```python
from build123d import *

# Parameters (mm, degrees)
SKETCH_1_W          = 100
SKETCH_1_H          = 5
EXTRUDE_1_DEPTH     = 8.8
SKETCH_2_W          = 5
SKETCH_2_H          = 10
EXTRUDE_2_DEPTH     = 8.8
SKETCH_3_W          = 5
SKETCH_3_H          = 10
EXTRUDE_3_DEPTH     = 8.8
SKETCH_4_W          = 5
SKETCH_4_H          = 5
EXTRUDE_4_DEPTH     = 8.8
SKETCH_5_W          = 5
SKETCH_5_H          = 5
EXTRUDE_5_DEPTH     = 8.8
SKETCH_6_W          = 0.3
SKETCH_6_H          = 5
CUT_EXTRUDE_1_DEPTH = 8.8
SKETCH_7_W          = 5
SKETCH_7_H          = 20.5
EXTRUDE_6_DEPTH     = 8.8
SKETCH_8_W          = 5
SKETCH_8_H          = 20.5
EXTRUDE_7_DEPTH     = 8.8
SKETCH_9_W          = 15
SKETCH_9_H          = 6
EXTRUDE_8_DEPTH     = 8.8
SKETCH_10_W         = 15
SKETCH_10_H         = 6
EXTRUDE_9_DEPTH     = 8.8
SKETCH_11_W         = 1.5
SKETCH_11_H         = 1.5
EXTRUDE_10_DEPTH    = 8.8
SKETCH_12_W         = 1.5
SKETCH_12_H         = 1.5
EXTRUDE_11_DEPTH    = 8.8
CUT_EXTRUDE_2_DEPTH = 1.8
SKETCH_15_W         = 1.5
SKETCH_15_H         = 1.5
CUT_EXTRUDE_3_DEPTH = 10
SKETCH_16_W         = 1.5
SKETCH_16_H         = 1.5
CUT_EXTRUDE_4_DEPTH = 10
SKETCH_17_W         = 7
SKETCH_17_H         = 6
EXTRUDE_12_DEPTH    = 5
SKETCH_18_W         = 7
SKETCH_18_H         = 6
EXTRUDE_13_DEPTH    = 5
SKETCH_19_W         = 7
SKETCH_19_H         = 6
EXTRUDE_14_DEPTH    = 1
SKETCH_20_W         = 7
SKETCH_20_H         = 6
EXTRUDE_15_DEPTH    = 1


with BuildPart() as part:
    # 草图1 → 凸台-拉伸1 (new body)
    with BuildSketch(Plane.XY):
        Rectangle(SKETCH_1_W, SKETCH_1_H)
    extrude(amount=EXTRUDE_1_DEPTH)

    # 草图2 → 凸台-拉伸2 (add)
    with BuildSketch(Plane(origin=(0, 0, 0), x_dir=(-1, 0, 0), z_dir=(0, 0, -1))):
        with Locations((-52.5, 2.5)):
            Rectangle(SKETCH_2_W, SKETCH_2_H)
    extrude(amount=-EXTRUDE_2_DEPTH)

    # 草图3 → 凸台-拉伸3 (add)
    with BuildSketch(Plane(origin=(0, 0, 0), x_dir=(-1, 0, 0), z_dir=(0, 0, -1))):
        with Locations((52.5, 2.5)):
            Rectangle(SKETCH_3_W, SKETCH_3_H)
    extrude(amount=-EXTRUDE_3_DEPTH)

    # 草图4 → 凸台-拉伸4 (add)
    with BuildSketch(Plane.XY.offset(8.8)):
        with Locations((-57.5, 5)):
            Rectangle(SKETCH_4_W, SKETCH_4_H)
    extrude(amount=-EXTRUDE_4_DEPTH)

    # 草图5 → 凸台-拉伸5 (add)
    with BuildSketch(Plane.XY.offset(8.8)):
        with Locations((57.5, 5)):
            Rectangle(SKETCH_5_W, SKETCH_5_H)
    extrude(amount=-EXTRUDE_5_DEPTH)

    # 草图6 → 切除-拉伸1 (cut)
    with BuildSketch(Plane.XY.offset(8.8)):
        with Locations((-50.15, 5)):
            Rectangle(SKETCH_6_W, SKETCH_6_H)
    extrude(amount=-CUT_EXTRUDE_1_DEPTH, mode=Mode.SUBTRACT)

    # 草图7 → 凸台-拉伸6 (add)
    with BuildSketch(Plane.XY.offset(8.8)):
        with Locations((-62.5, 12.75)):
            Rectangle(SKETCH_7_W, SKETCH_7_H)
    extrude(amount=-EXTRUDE_6_DEPTH)

    # 草图8 → 凸台-拉伸7 (add)
    with BuildSketch(Plane.XY.offset(8.8)):
        with Locations((62.5, 12.75)):
            Rectangle(SKETCH_8_W, SKETCH_8_H)
    extrude(amount=-EXTRUDE_7_DEPTH)

    # 草图9 → 凸台-拉伸8 (add)
    with BuildSketch(Plane.XY.offset(8.8)):
        with Locations((-57.5, 26)):
            Rectangle(SKETCH_9_W, SKETCH_9_H)
    extrude(amount=-EXTRUDE_8_DEPTH)

    # 草图10 → 凸台-拉伸9 (add)
    with BuildSketch(Plane.XY.offset(8.8)):
        with Locations((57.5, 26)):
            Rectangle(SKETCH_10_W, SKETCH_10_H)
    extrude(amount=-EXTRUDE_9_DEPTH)

    # 草图11 → 凸台-拉伸10 (add)
    with BuildSketch(Plane.XY.offset(8.8)):
        with Locations((-50.75, 22.25)):
            Rectangle(SKETCH_11_W, SKETCH_11_H)
    extrude(amount=-EXTRUDE_10_DEPTH)

    # 草图12 → 凸台-拉伸11 (add)
    with BuildSketch(Plane.XY.offset(8.8)):
        with Locations((50.75, 22.25)):
            Rectangle(SKETCH_12_W, SKETCH_12_H)
    extrude(amount=-EXTRUDE_11_DEPTH)

    # 草图14 → 切除-拉伸2 (cut)
    with BuildSketch(Plane.XY.offset(8.8)):
        Polygon((-51.5, 23), (-51.5, 21.5), (-50, 21.5), (-50, 29), (-65, 29), (-65, 2.5), (-55, 2.5), (-55, -2.5), (55, -2.5), (55, 2.5), (65, 2.5), (65, 29), (50, 29), (50, 21.5), (51.5, 21.5), (51.5, 23), (60, 23), (60, 7.5), (50, 7.5), (50, 2.5), (-50.3, 2.5), (-50.3, 7.5), (-60, 7.5), (-60, 23), align=None)
    extrude(amount=-CUT_EXTRUDE_2_DEPTH, mode=Mode.SUBTRACT)

    # 草图15 → 切除-拉伸3 (cut)
    with BuildSketch(Plane.XY.offset(7)):
        with Locations((-50.75, 22.25)):
            Rectangle(SKETCH_15_W, SKETCH_15_H)
    extrude(amount=-CUT_EXTRUDE_3_DEPTH, mode=Mode.SUBTRACT)

    # 草图16 → 切除-拉伸4 (cut)
    with BuildSketch(Plane.XY.offset(7)):
        with Locations((50.75, 22.25)):
            Rectangle(SKETCH_16_W, SKETCH_16_H)
    extrude(amount=-CUT_EXTRUDE_4_DEPTH, mode=Mode.SUBTRACT)

    # 草图17 → 凸台-拉伸12 (add)
    with BuildSketch(Plane(origin=(-50, 0, 0), x_dir=(0, 0, -1), z_dir=(1, 0, 0))):
        with Locations((-3.5, 26)):
            Rectangle(SKETCH_17_W, SKETCH_17_H)
    extrude(amount=EXTRUDE_12_DEPTH)

    # 草图18 → 凸台-拉伸13 (add)
    with BuildSketch(Plane.ZY.offset(-50)):
        with Locations((3.5, 26)):
            Rectangle(SKETCH_18_W, SKETCH_18_H)
    extrude(amount=EXTRUDE_13_DEPTH)

    # 草图19 → 凸台-拉伸14 (add)
    with BuildSketch(Plane(origin=(-45, 0, 0), x_dir=(0, 0, -1), z_dir=(1, 0, 0))):
        with Locations((-3.5, 26)):
            Rectangle(SKETCH_19_W, SKETCH_19_H)
    extrude(amount=EXTRUDE_14_DEPTH)

    # 草图20 → 凸台-拉伸15 (add)
    with BuildSketch(Plane.ZY.offset(-45)):
        with Locations((3.5, 26)):
            Rectangle(SKETCH_20_W, SKETCH_20_H)
    extrude(amount=EXTRUDE_15_DEPTH)


solid = part.part
```
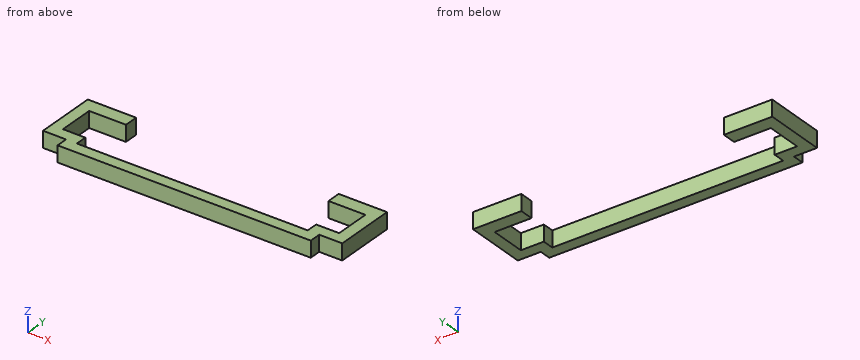
Work out the finished part from the listing and answer in its coordinate system (mm). Give positions to 0.01 mm unless a question says otherwise; leave off trailing zeros. Order: outer loops, then holes, each group sorted by start corner. A loop starts at its lowest first (then second) coordinate and runs counter-clockwise, first axis right, second up. Notation, with made-up numbers: M -1,12.5 L 42,12.5 A23 cw 42,21.5 Z; hole C 17.25,58 d2. An arc over 180 degrees is marked long. Return JSON: item names as keys, results as strings.
1) Straight lines are drawn through the part: line 1 along X through (y, z) = (17, 1.5); line 2 along X through (y, z) = (5.5, 1.5); line 3 along Y through (x, z) = (47.5, 5.25). For each, find the intervals that lie inside material, in ascending order. Write a range as [from, to].
Resolved:
{"line 1": "[-65, -60], [60, 65]", "line 2": "[-65, -50.3], [50, 65]", "line 3": "[-2.5, 2.5], [23, 29]"}
2) Section B-B, the plane x = 56.5 is taken. Write down the section's boundary in (y, z), plus the area to 3 significant figures.
Resolved:
{"outline": "M 2.5,0 L 7.5,0 L 7.5,7 L 2.5,7 Z; M 23,0 L 29,0 L 29,7 L 23,7 Z", "area": "77.0 mm^2"}
3) Section C-C, the plane z = 3.5 is taken. Write down the section's boundary in (x, y).
Resolved:
{"outline": "M -65,2.5 L -55,2.5 L -55,-2.5 L 55,-2.5 L 55,2.5 L 65,2.5 L 65,29 L 44,29 L 44,23 L 60,23 L 60,7.5 L 50,7.5 L 50,2.5 L -50.3,2.5 L -50.3,7.5 L -60,7.5 L -60,23 L -44,23 L -44,29 L -65,29 Z"}
4) Each of these flat-tipped pins is pushed along its axis until it touches: pin 1 (3 mm diameter, centred on x = 44, y = 5.5, fed in from -Z) (3 decimals); pin 2 (3.5 mm diameter, centred on x = 59.5, z = 3, fed in from -Y); pin 3 (12 mm diameter, centred on x = 13.5, y = 7, fed in from -Z); pin 4 (2 mm diameter, centred on x = 16.5, z = 2.5, fed in from +Y). Where does it stop, or does it pass through?
Resolved:
{"pin 1": "through", "pin 2": "y = 2.5", "pin 3": "z = 0", "pin 4": "y = 2.5"}
5) Section D-D, the plane x = -19.5 is taken. Write down the section's boundary in (y, z), plus the area to 3 significant figures.
Resolved:
{"outline": "M -2.5,0 L 2.5,0 L 2.5,7 L -2.5,7 Z", "area": "35.0 mm^2"}
6) Section A-A, the plane y = 5.5 is taken. Write down the section's boundary in (x, z), plus the area to 3 significant figures.
Resolved:
{"outline": "M -65,0 L -50.3,0 L -50.3,7 L -65,7 Z; M 50,0 L 65,0 L 65,7 L 50,7 Z", "area": "208 mm^2"}
